Geometry check sheet. Reference: the model listing, model coordinates, mm. Round coordinates to 2 decimals unless told otherwise and drop trailing zeros. Write each loop counter-clockwise with the first axis right and the second up, starting at its lowest first coordinate (ties: lowest second). Pieces come first, ordered by that corner, then holes. Notation, with made-up numbers: (35, 26.25) - (86, 26.25) arc R26 cw to (86, 42.25) - close; hole circle Ø5 at (-24, 24.25). An arc over 180 degrees is marked (long way). Return JSON: item names as keys, results as strings.
```python
from build123d import *

# Parameters (mm, degrees)
ESQUISSE1_W        = 48
ESQUISSE1_H        = 50
BOSS_EXTRU_1_DEPTH = 70
ESQUISSE2_R        = 2.5
ESQUISSE2_R_2      = 0.6
BOSS_EXTRU_2_DEPTH = 20


with BuildPart() as part:
    # Esquisse1 → Boss.-Extru.1 (new, symmetric)
    with BuildSketch(Plane.XY):
        Rectangle(ESQUISSE1_W, ESQUISSE1_H)
    extrude(amount=BOSS_EXTRU_1_DEPTH, both=True)

    # Esquisse2 → Boss.-Extru.2 (add)
    with BuildSketch(Plane.XY.offset(70)):
        with Locations((-19.03905832, 22)):
            Circle(ESQUISSE2_R)
        with Locations((-13.03905832, 22)):
            Circle(ESQUISSE2_R)
        with Locations((15.464385939, 23.480295556)):
            Circle(ESQUISSE2_R_2)
        with Locations((16.764385939, 23.480295556)):
            Circle(ESQUISSE2_R_2)
        with Locations((18.064385939, 23.480295556)):
            Circle(ESQUISSE2_R_2)
        with Locations((19.364385939, 23.480295556)):
            Circle(ESQUISSE2_R_2)
        with Locations((14.164385939, 23.480295556)):
            Circle(ESQUISSE2_R_2)
    extrude(amount=BOSS_EXTRU_2_DEPTH)


solid = part.part
```
(1) Section check A-A, the plane x = -7. Enter the section's corners in (y, z), plus the area to 3 significant figures.
Response values:
{"outline": "(-25, -70) - (25, -70) - (25, 70) - (-25, 70) - close", "area": "7,000 mm^2"}
(2) Gauge pin test, flat end, axial feed: pin 1 (10 mm diameter, centred on x = 10, y = 2.5, fed in from +Z). Record the tip position at first contact, or that the pin passes through.
Response values:
{"pin 1": "stops at z = 70"}
(3) Material ranges on line 1 along Z through (x, y) = (14, 6), recorded low to high. Write a range as [from, to].
Response values:
{"line 1": "z = [-70, 70]"}
(4) Section check B-B, the plane y = -17. Enter the section's corners in (x, z).
Response values:
{"outline": "(-24, -70) - (24, -70) - (24, 70) - (-24, 70) - close"}
(5) Release check for a two-part mould opening along X. For faces 1 (the face through (0, 25, 1)), 2 (the face through (-13.36, 24.48, 79.86)), 3 (the face through (-24, 0, 1)), 4 (the face through (-19.36, 24.48, 79.86)) record: pulls with the +X half, pulls with the -X half, needs draft (parallel to the pull), parting line crosses it, or undercut.
Response values:
{"face 1": "needs draft", "face 2": "undercut", "face 3": "pulls with the -X half", "face 4": "undercut"}
